Geometry: final body of the model. Coordinates: model frame, mm. Face numbers are marked on the shaded views. A direction names the side the tool comes from. Round coordinates to 2 decimals unless told otherwise and drop trailing zeros. Loops run counter-clockwise (first coordinate to the right, second up) from the corner with the lowest first, then second, coordinate; pieces in that order, holes last. Notation, with made-up numbers: (-1, 73) -> (5, 73) arc R23 ccw to (5, 84) -> close; hole circle Ø4 at (78, 1.5). An arc over 180 degrees is marked (long way). Answer in a Markdown table with one row per item.
```python
from build123d import *

# Parameters (mm, degrees)
SKETCH1_W           = 8
SKETCH1_H           = 9.6
BOSS_EXTRUDE1_DEPTH = 16
SKETCH4_W           = 4.8
SKETCH4_H           = 12.8
CUT_EXTRUDE1_DEPTH  = 8
SKETCH5_R           = 2.4
BOSS_EXTRUDE2_DEPTH = 1.6
BOSS_EXTRUDE3_DEPTH = 4.8
SKETCH7_R           = 2.5
CUT_EXTRUDE2_DEPTH  = 3.5
CUT_EXTRUDE3_DEPTH  = 4.5
SKETCH9_R           = 3.25
SKETCH9_R_2         = 2.5
BOSS_EXTRUDE4_DEPTH = 1.6
SKETCH10_W          = 1.6
SKETCH10_H          = 6.5
CUT_EXTRUDE4_DEPTH  = 1


with BuildPart() as part:
    # Sketch1 → Boss-Extrude1 (new body)
    with BuildSketch(Plane.XY):
        with Locations((4, 4.8)):
            Rectangle(SKETCH1_W, SKETCH1_H)
    extrude(amount=BOSS_EXTRUDE1_DEPTH)

    # Sketch4 → Cut-Extrude1 (cut)
    with BuildSketch(Plane.XZ):
        with Locations((4, 8)):
            Rectangle(SKETCH4_W, SKETCH4_H)
    extrude(amount=-CUT_EXTRUDE1_DEPTH, mode=Mode.SUBTRACT)

    # Sketch5 → Boss-Extrude2 (add)
    with BuildSketch(Plane(origin=(0, 9.6, 0), x_dir=(1, 0, 0), z_dir=(0, 1, 0))):
        with Locations((4, -12)):
            Circle(SKETCH5_R)
        with Locations((4, -4)):
            Circle(SKETCH5_R)
    extrude(amount=BOSS_EXTRUDE2_DEPTH)

    # Sketch6 → Boss-Extrude3 (add)
    with BuildSketch(Plane.ZY.offset(-6.4)):
        with BuildLine():
            ThreePointArc((9.802775638, 8), (8, 8.5), (6.197224362, 8))
            Line((6.197224362, 8), (9.802775638, 8))
        make_face()
        with BuildLine():
            Line((9.802775638, 8), (6.197224362, 8))
            ThreePointArc((6.197224362, 8), (6.276589824, 1.953714169), (11.5, 5))
            ThreePointArc((11.5, 5), (11.046285831, 6.723410176), (9.802775638, 8))
        make_face()
    extrude(amount=BOSS_EXTRUDE3_DEPTH)

    # Sketch7 → Cut-Extrude2 (cut)
    with BuildSketch(Plane.ZY):
        with Locations((8, 5)):
            Circle(SKETCH7_R)
    extrude(amount=-CUT_EXTRUDE2_DEPTH, mode=Mode.SUBTRACT)

    # Sketch8 → Cut-Extrude3 (cut)
    with BuildSketch(Plane.ZY.offset(-3.5)):
        with BuildLine():
            ThreePointArc((8.5, 7.449489743), (8, 7.5), (7.5, 7.449489743))
            Line((7.5, 7.449489743), (7.5, 2.550510257))
            ThreePointArc((7.5, 2.550510257), (8, 2.5), (8.5, 2.550510257))
            Line((8.5, 2.550510257), (8.5, 7.449489743))
        make_face()
    extrude(amount=-CUT_EXTRUDE3_DEPTH, mode=Mode.SUBTRACT)

    # Sketch9 → Boss-Extrude4 (add)
    with BuildSketch(Plane.ZY):
        with Locations((8, 5)):
            Circle(SKETCH9_R)
        with Locations((8, 5)):
            Circle(SKETCH9_R_2, mode=Mode.SUBTRACT)
    extrude(amount=BOSS_EXTRUDE4_DEPTH)

    # Sketch10 → Cut-Extrude4 (cut)
    with BuildSketch(Plane(origin=(0, 8.25, 0), x_dir=(1, 0, 0), z_dir=(0, 1, 0))):
        with Locations((-0.8, -8)):
            Rectangle(SKETCH10_W, SKETCH10_H)
    extrude(amount=-CUT_EXTRUDE4_DEPTH, mode=Mode.SUBTRACT)


solid = part.part
```
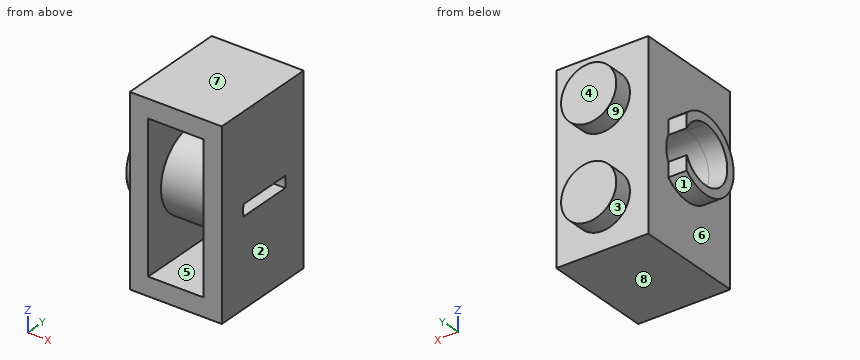
Item 1: Section query B-B, the plane y = 3.25. Output: boundary loops of the cut face in (x, z).
Ans:
| item | result |
|---|---|
| outline | (-1.6, 5.26) -> (0, 5.26) -> (0, 0) -> (8, 0) -> (8, 7.5) -> (3.5, 7.5) -> (3.5, 6.21) -> (-1.6, 6.21) -> close; (-1.6, 9.79) -> (3.5, 9.79) -> (3.5, 8.5) -> (8, 8.5) -> (8, 16) -> (0, 16) -> (0, 10.74) -> (-1.6, 10.74) -> close; hole (1.6, 1.6) -> (6.4, 1.6) -> (6.4, 4.97) -> (1.6, 4.97) -> close; hole (1.6, 11.03) -> (6.4, 11.03) -> (6.4, 14.4) -> (1.6, 14.4) -> close |
Item 2: Section query A-A, the plane z = 8. Output: boundary loops of the cut face in (x, y).
Ans:
| item | result |
|---|---|
| outline | (-1.6, 1.75) -> (0, 1.75) -> (0, 0) -> (1.6, 0) -> (1.6, 1.5) -> (6.4, 1.5) -> (6.4, 0) -> (8, 0) -> (8, 2.5) -> (-1.6, 2.5) -> close; (0, 7.5) -> (8, 7.5) -> (8, 9.6) -> (0, 9.6) -> close |
Item 3: Set-up query: the marked faces 1, 2, 3, 4 and 5. Return all of +Z, -Z, +X, -X, +Y, -Y with unobstructed straight access to the full face (end or side cutting, diameter ignored); none if empty.
Ans:
| item | result |
|---|---|
| face 1 | -X |
| face 2 | +Z, -Z, +X, +Y, -Y |
| face 3 | +Y |
| face 4 | +Z, -Z, +X, -X, +Y |
| face 5 | -Y |
Item 4: Ray query, L1, parallel to Z at x = 5, y = 5; L2, parallel to Z at x = 6, y = 2; L3, parallel to Y at x = 4.25, z = 8. Return the intervals inside material, ascending.
Ans:
| item | result |
|---|---|
| L1 | 0 to 1.6, 4.5 to 7.5, 8.5 to 11.5, 14.4 to 16 |
| L2 | 0 to 1.6, 6.2 to 9.8, 14.4 to 16 |
| L3 | 1.5 to 2.5, 7.5 to 9.6 |
Item 5: Section query D-D, the plane x = 4. Output: boundary loops of the cut face in (y, z).
Ans:
| item | result |
|---|---|
| outline | (0, 0) -> (9.6, 0) -> (9.6, 1.6) -> (11.2, 1.6) -> (11.2, 6.4) -> (9.6, 6.4) -> (9.6, 9.6) -> (11.2, 9.6) -> (11.2, 14.4) -> (9.6, 14.4) -> (9.6, 16) -> (0, 16) -> (0, 14.4) -> (8, 14.4) -> (8, 9.8) arc R3.5 ccw (long way) to (8, 6.2) -> (8, 1.6) -> (0, 1.6) -> close; hole (2.55, 7.5) -> (7.45, 7.5) arc R2.5 ccw to (7.45, 8.5) -> (2.55, 8.5) arc R2.5 ccw to start |
Item 6: First-contact query: P1, Ø1, axis at x = -1, z = 6.5, coming from the +Y side; P2, Ø2.5, axis at x = 5, z = 4, coming from the -Y side; P3, Ø3, axis at x = 3.5, z = 12, coming from the -Y side. Flat tips, straight axial feed; report the tip coordinate or a pass-through.
Ans:
| item | result |
|---|---|
| P1 | y = 7.25 |
| P2 | y = 2.83 |
| P3 | y = 2.55 |
Item 7: Mould query, pull axis Z, two halves, no side actions, for the marked faces 6, 7, 8 and 9. Classes: released by +Z, released by -Z, zero draft, split by the parting line, or undercut.
Ans:
| item | result |
|---|---|
| face 6 | zero draft |
| face 7 | released by +Z |
| face 8 | released by -Z |
| face 9 | undercut |
Item 8: Section query C-C, the plane y = 1.25. Output: boundary loops of the cut face in (x, z), and give its area (3 significant figures).
Ans:
| item | result |
|---|---|
| outline | (0, 0) -> (8, 0) -> (8, 16) -> (0, 16) -> close; hole (1.6, 1.6) -> (6.4, 1.6) -> (6.4, 14.4) -> (1.6, 14.4) -> close |
| area | 66.6 mm2 |
